Geometry check sheet. Reference: the model listing, model coordinates, mm. A direction names the side the tool comes from. Give positions to 0.01 mm unless a question says otherwise; leave off trailing zeros. Write each loop counter-clockwise with the first axis right and the second up, starting at its lowest first coordinate (ties: lowest second). Pieces come first, ordered by that corner, then holes.
(1) Thickness scan on line 1 along Z through (x, y) = (4, 12.75); line 2 along X through (y, z) = (4, 0); line 3 along X through (y, z) = (2.25, -4.75). Record the ranges inside material, lowest first.
(2) Depth check by flat-ended pin: P1, Ø4.5, axis at x = -7, y = 8, coming from the +Z side; P2, Ø2, axis at x = -4, y = 8.5, coming from the -Z side; P3, Ø2.5, axis at x = 8.23, z = -4.75, coming from the -Y side. Enter the tip coordinate at first touch or a pass-through.
(3) Cross-section at A-A (x = 0). Record the boundary of the cut face in (y, z) (3 decimals).
(4) Cross-section at C-C (y = 5.75). Record the boundary of the cut face in (x, z).
(5) Mould release check, pull along X, two halves, no side actions. Record for faces 1 (the flat face through (3.2, 0, -3.2)), 2 (the cylindrical face through (10.277, 3.204, -4.295)), 3 (the flat face through (0, 11.15, 7)): +X half, -X half, draft (parallel to the pull), parting line (faces both ways), or undercut.
(6) Tool access check on faces 4 (the cylindrical face through (-10.31, 3.2, -4.48)), 5 (the flat face through (8, 7, 0)), 6 (the flat face through (-12, 14.15, 5)). Record the directions out of +Z, -Z, +X, -X, +Y, -Y that give a thin tool (end or side, any length) a straight path to the whole face; none if there is none.
(7) Cross-section at B-B (z = 0). Record the boundary of the cut face in (x, y) (3 decimals).
```python
from build123d import *
from build123d.topology import SkipClean

# Parameters (mm, degrees)
SKETCH1_R                       = 15
BOSS_EXTRUDE1_DEPTH             = 7
SKETCH2_R                       = 4.2
CUT_EXTRUDE1_DEPTH              = 7
BOSS_EXTRUDE2_DEPTH             = 4.15
SKETCH1_5_R                     = 2.1
CUT_EXTRUDE2_DEPTH              = 6.5
SKETCH6_R                       = 15
SKETCH6_R_2                     = 12.775
BOSS_EXTRUDE3_DEPTH             = 3
BOSS_EXTRUDE3_DIRECTION_2_REACH = 25.965
FILLET1_R                       = 1.5


with BuildPart() as part:
    # Sketch1 → Boss-Extrude1 (new body)
    with BuildSketch(Plane(origin=(0, 0, 0), x_dir=(1, 0, 0), z_dir=(0, 1, 0))):
        with Locations(Location((0, 0, 0), (0, 0, 270))):
            Circle(SKETCH1_R)
    extrude(amount=BOSS_EXTRUDE1_DEPTH)

    # Sketch2 → Cut-Extrude1 (cut)
    with BuildSketch(Plane(origin=(0, 0, 0), x_dir=(1, 0, 0), z_dir=(0, 1, 0))):
        with Locations(Location((0, 0, 0), (0, 0, 270))):
            Circle(SKETCH2_R)
    extrude(amount=CUT_EXTRUDE1_DEPTH, mode=Mode.SUBTRACT)

    # Sketch5 → Boss-Extrude2 (add)
    with SkipClean():  # the faces are left unmerged after this step: merging them gives an invalid solid
        with BuildSketch(Plane(origin=(0, 7, 0), x_dir=(1, 0, 0), z_dir=(0, 1, 0))):
            with BuildLine():
                ThreePointArc((14.456832, 4), (0, 15), (-14.456832, 4))
                Line((-14.456832, 4), (-1.280625, 4))
                ThreePointArc((-1.280625, 4), (0, 4.2), (1.280625, 4))
                Line((1.280625, 4), (14.456832, 4))
            make_face()
            with BuildLine():
                Line((-1.280625, -4), (-14.456832, -4))
                ThreePointArc((-14.456832, -4), (0, -15), (14.456832, -4))
                Line((14.456832, -4), (1.280625, -4))
                ThreePointArc((1.280625, -4), (0, -4.2), (-1.280625, -4))
            make_face()
        extrude(amount=BOSS_EXTRUDE2_DEPTH)

    # Sketch1<5> → Cut-Extrude2 (cut)
    with SkipClean():  # the faces are left unmerged after this step: merging them gives an invalid solid
        with BuildSketch(Plane(origin=(0, 0, 0), x_dir=(1, 0, 0), z_dir=(0, 1, 0))):
            with Locations(Location((0, -9.5, 0), (0, 0, 90))):
                Circle(SKETCH1_5_R)
            with Locations(Location((-8.227241, 4.75, 0), (0, 0, 90))):
                Circle(SKETCH1_5_R)
            with Locations(Location((8.227241, 4.75, 0), (0, 0, 90))):
                Circle(SKETCH1_5_R)
        extrude(amount=CUT_EXTRUDE2_DEPTH, mode=Mode.SUBTRACT)

    # Sketch6 → Boss-Extrude3 (add)
    with SkipClean():  # the faces are left unmerged after this step: merging them gives an invalid solid
        with BuildSketch(Plane(origin=(0, 11.15, 0), x_dir=(1, 0, 0), z_dir=(0, 1, 0))):
            with Locations(Location((0, 0, 0), (0, 0, 270))):
                Circle(SKETCH6_R)
            with Locations(Location((0, 0, 0), (0, 0, 270))):
                Circle(SKETCH6_R_2, mode=Mode.SUBTRACT)
        extrude(amount=BOSS_EXTRUDE3_DEPTH)

    # Boss-Extrude3 direction 2: up to this face of the body (flat: up to its plane)
    boss_extrude3_direction_2_end = Plane(part.part.faces().sort_by_distance((-9.095084, 7, 0))[0])
    # Sketch6 → Boss-Extrude3 direction 2 (add, up to the picked face)
    with BuildSketch(Plane(origin=(0, 11.15, 0), x_dir=(1, 0, 0), z_dir=(0, 1, 0)), mode=Mode.PRIVATE) as boss_extrude3_direction_2_sk1:
        with Locations(Location((0, 0, 0), (0, 0, 270))):
            Circle(SKETCH6_R)
        with Locations(Location((0, 0, 0), (0, 0, 270))):
            Circle(SKETCH6_R_2, mode=Mode.SUBTRACT)
    boss_extrude3_direction_2_tool1 = split(extrude(boss_extrude3_direction_2_sk1.sketch, amount=-BOSS_EXTRUDE3_DIRECTION_2_REACH, mode=Mode.PRIVATE), bisect_by=boss_extrude3_direction_2_end, keep=Keep.BOTH, mode=Mode.PRIVATE)
    add(boss_extrude3_direction_2_tool1.solids().sort_by(Axis((0, 11.15, -14.575736), (0, -1, 0)))[0])

    # Fillet1
    fillet1_edges = [part.edges().sort_by_distance(p)[0] for p in [
        (0, 0, -15),
        (0, 14.15, -15),
    ]]
    fillet(fillet1_edges, radius=FILLET1_R)


solid = part.part
```
Reply:
1. line 1: z = -14.45 to -12.13, 12.13 to 14.45
1. line 2: x = -15 to -4.2, 4.2 to 15
1. line 3: x = -14.23 to -10.33, -6.13 to 6.13, 10.33 to 14.23
2. P1: stops at z = 14.23
2. P2: stops at z = -14.7
2. P3: stops at y = 6.5
3. outline: (0, -13.5) arc R1.5 ccw to (1.5, -15) - (12.65, -15) arc R1.5 ccw to (14.15, -13.5) - (14.15, -12.775) - (11.15, -12.775) - (11.15, -4.2) - (0, -4.2) - close; (0, 4.2) - (11.15, 4.2) - (11.15, 12.775) - (14.15, 12.775) - (14.15, 13.5) arc R1.5 ccw to (12.65, 15) - (1.5, 15) arc R1.5 ccw to (0, 13.5) - (0, 11.6) - (6.5, 11.6) - (6.5, 7.4) - (0, 7.4) - close
4. outline: circle Ø30 at (0, 0); hole circle Ø4.2 at (-8.23, -4.75); hole circle Ø8.4 at (0, 0); hole circle Ø4.2 at (0, 9.5); hole circle Ø4.2 at (8.23, -4.75)
5. face 1: draft
5. face 2: undercut
5. face 3: undercut
6. face 4: -Y
6. face 5: +Y
6. face 6: +Z, -Z, +X, -X, +Y
7. outline: (-15, 1.5) arc R1.5 ccw to (-13.5, 0) - (-4.2, 0) - (-4.2, 7) - (-12.775, 7) - (-12.775, 14.15) - (-13.5, 14.15) arc R1.5 ccw to (-15, 12.65) - close; (4.2, 0) - (13.5, 0) arc R1.5 ccw to (15, 1.5) - (15, 12.65) arc R1.5 ccw to (13.5, 14.15) - (12.775, 14.15) - (12.775, 7) - (4.2, 7) - close
